Input: dimensioned drawing with shaded views. Units: mm. Origin: part minimum x, y, z. Coordinates: 2 decimals unless noted, no trailing zeros. Order: outer loops, then holes, each group sorted by start corner. A loop starts at its lowest first (then second) coordinate and runs counter-clockwise, first axis right, second up. Notation, with made-up numbers: (18.5, -5) - (77.5, -5) arc R30 ccw to (77.5, 32) - close; hole circle Ø10 at (16.25, 89.25). An arc over 180 degrees is marked (long way). One line per question, with ' | ' between items. Start each with the question number.
(1) Section C-C (y = 10). Return the cut outline in (x, z).
(2) Section B-B (z = 2). Count the separate pieces of the cut face and the enclosed holes in it, then the cut area to 3 significant figures.
(3) Section A-A (x = 10). Return the cut outline in (y, z).
(4) Contact query for flat-ended pins moving along their axis: P1, Ø1.5, axis at y = 6, z = 1.5, coming from the +X side; P2, Ø1.5, axis at x = 47.5, z = 1, coming from the -Y side; P3, Ø1.5, axis at y = 35, z = 2, coming from the -X side. Output: stop coordinate, or through.
(5) Line query: line 1 along Y through (x, z) = (30, 0.75); line 2 along X through (y, z) = (13, 1.3); line 3 along Y through (x, z) = (14.5, 0.65). Output: solid intervals per line, ascending.
(6) Section D-D (y = 18). Return the cut outline in (x, z).
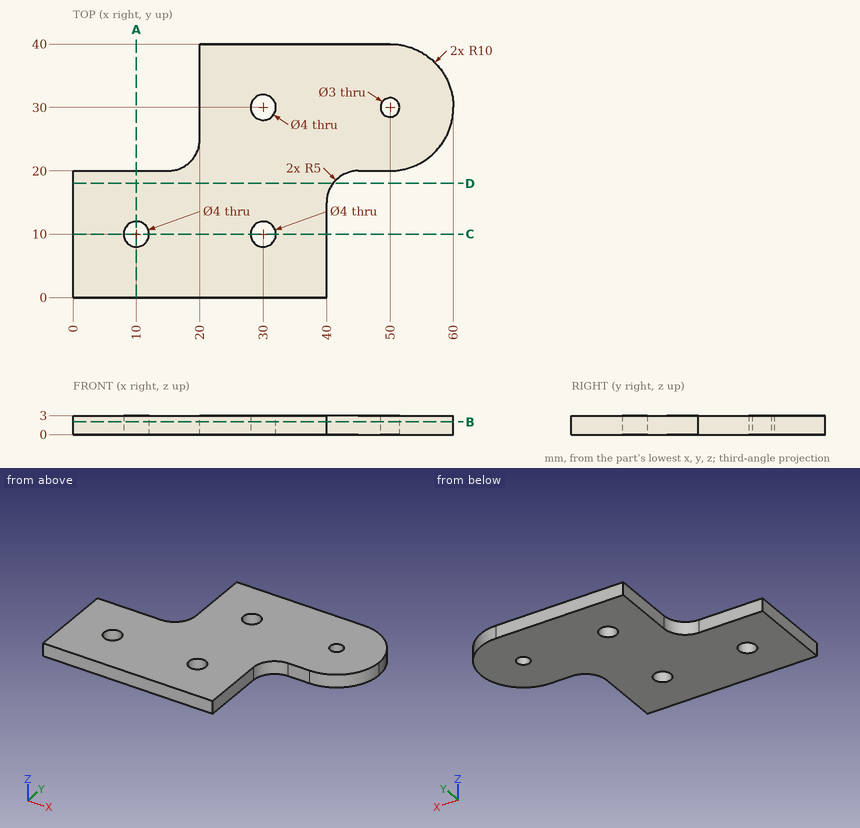
Response values:
1) outline: (0, 0) - (8, 0) - (8, 3) - (0, 3) - close; (12, 0) - (28, 0) - (28, 3) - (12, 3) - close; (32, 0) - (40, 0) - (40, 3) - (32, 3) - close
2) separate pieces: 1 | enclosed holes: 4 | area: 1,520 mm²
3) outline: (0, 0) - (8, 0) - (8, 3) - (0, 3) - close; (12, 0) - (20, 0) - (20, 3) - (12, 3) - close
4) P1: stops at x = 40 | P2: stops at y = 20 | P3: stops at x = 20
5) line 1: y = 0 to 8, 12 to 28, 32 to 40 | line 2: x = 0 to 40 | line 3: y = 0 to 20
6) outline: (0, 0) - (41, 0) - (41, 3) - (0, 3) - close
